Verification items for the finished model (mm, model axes). A direction names the side the tool comes from. Coordinates: 2 decimals unless noted, no trailing zeros. Order: outer loops, then holes, each group sorted by start corner. A loop starts at its lowest first (then second) coordinate and runs counter-clockwise, first axis right, second up. Notation, with made-up numbers: M -32,-6.75 L 16,-6.75 A31 ccw 16,25.25 Z; hole C -40,-23 d8. An arc over 180 degrees is marked long. Answer as a JSON object with one key per item and string values. Group by question number.
(1) Material ranges on line 1 (X direction, y = -21.5, z = -60) (3 decimals); line 2 (Z direction, x = -57, y = -12.75) (3 decimals); line 3 (Y direction, x = 48.5, z = 55), recorded low to high.
(2) Gauge pin test, flat end, axial feed: pin 1 Ø6 at (x, z) = (-25.5, 2) entering from -Y. Record the tip position at first contact, or that the pin passes through.
(3) Mould release check, pull along X, two halves, no side actions. Record for faces 3 (the face through (79.375, -10, 1)), 4 (the face through (-76.835, -11, 1)), 5 (the face through (-1, 2.54, -1)), 6 (the face through (-79.375, -10, 1)): released by +X, released by -X, zero draft, split by the parting line, or undercut.
(4) Cross-section at B-B (x = -14.5). Enter the section's corners in (y, z) (3 decimals).
(5) Cross-section at A-A (y = -14.75). Enter the section's corners in (x, z) (3 decimals), plus the area to 3 significant figures.
(6) Access from +Z, -Z, +X, -X, +Y, -Y to the whole of each face (thin tool, end or side, straight path). Record for faces 1 (the face through (-1, -10, -92.075)), 2 (the face through (-1, -11, 89.535)).
(7) Cross-section at C-C (z = -42). Enter the section's corners in (x, y) (3 decimals).
from build123d import *

# Parameters (mm, degrees)
SKETCH1_W           = 158.75
SKETCH1_H           = 184.15
BOSS_EXTRUDE1_DEPTH = 25.4
SHELL1_T            = -2.54


with BuildPart() as part:
    # Sketch1 → Boss-Extrude1 (new body)
    with BuildSketch(Plane(origin=(0, 2.54, 0), x_dir=(1, 0, 0), z_dir=(0, 1, 0))):
        Rectangle(SKETCH1_W, SKETCH1_H)
    extrude(amount=-BOSS_EXTRUDE1_DEPTH)

    # Shell1
    shell1_openings = [part.faces().sort_by_distance(p)[0] for p in [
        (0, -22.86, 0),
    ]]
    offset(amount=SHELL1_T, openings=shell1_openings, kind=Kind.INTERSECTION)


solid = part.part
Taken from the geometry:
{
 "1": {"line 1": "x = -79.375 to -76.835, 76.835 to 79.375", "line 2": "z = -92.075 to -89.535, 89.535 to 92.075", "line 3": "y = 0 to 2.54"},
 "2": {"pin 1": "stops at y = 0"},
 "3": {"face 3": "released by +X", "face 4": "undercut", "face 5": "zero draft", "face 6": "released by -X"},
 "4": {"outline": "M -22.86,-92.075 L 2.54,-92.075 L 2.54,92.075 L -22.86,92.075 L -22.86,89.535 L 0,89.535 L 0,-89.535 L -22.86,-89.535 Z"},
 "5": {"outline": "M -79.375,-92.075 L 79.375,-92.075 L 79.375,92.075 L -79.375,92.075 Z; hole M -76.835,-89.535 L 76.835,-89.535 L 76.835,89.535 L -76.835,89.535 Z", "area": "1,720 mm²"},
 "6": {"face 1": "-Z, +X, -X, +Y, -Y", "face 2": "-Y"},
 "7": {"outline": "M -79.375,-22.86 L -76.835,-22.86 L -76.835,0 L 76.835,0 L 76.835,-22.86 L 79.375,-22.86 L 79.375,2.54 L -79.375,2.54 Z"}
}
